Read the model definition and answer for the solid it produces. Units are mm, in the model's axes. A direction names the side the tool comes from. Coordinates: 2 decimals unless noted, no trailing zeros. Write each loop counter-clockwise with the first axis right and the second up, starting at its lowest first coordinate (ties: lowest second). Pieces come first, ordered by that corner, then holes.
(1) The part is cut by section B-B, the plane x = 89. Determine the outline of the cut face in (y, z).
(2) Which of the six approach directions +Z, -Z, +X, -X, +Y, -Y give full straight-line access (tool end or side, diameter ignored) to faces 4 (the flat face through (64, 34, 8)), 5 (the cylindrical face through (112.48, 60, 3.67)), 6 (the cylindrical face through (119.96, 38.81, 3.94))?
(3) Determine the mould class of faces 1 (the cylindrical face through (6.467, 1.862, 3.944)), 2 (the cylindrical face through (22.11, 60, 5.34)), 3 (the flat face through (20, 49.862, 4)) for opening direction Y: pulls with the +Y half, pulls with the -Y half, needs draft (parallel to the pull), parting line crosses it, or undercut.
(4) Given pin 1 (4.5 mm diameter, centred on x = 50, z = 4, fed in from +Y), flat-ended and moving along its own axis, determine where the tip first touches the part or whether it passes through.
(5) The part is cut by section C-C, the plane z = 4. State how many separate pieces and enclosed holes the cut face has, and give its area (3 significant figures).
(6) The part is cut by section A-A, the plane x = 123.5. Determine the outline of the cut face in (y, z), and give its area (3 significant figures).
(7) Straight lines are drawn through the part: line 1 along Y through (x, z) = (65, 2.5); line 2 along X through (y, z) = (7.5, 3.5); line 3 along X through (y, z) = (57.75, 4). For each, find the intervals that lie inside material, in ascending order.
(8) The part is cut by section D-D, the plane x = 50. Determine the outline of the cut face in (y, z), and give its area (3 significant figures).
```python
from build123d import *

# Parameters (mm, degrees)
BOSS_EXTRU_1_DEPTH       = 8
ESQUISSE2_W              = 5.5
ESQUISSE2_H              = 8
ESQUISSE2_W_2            = 6
ENL_V_MAT_EXTRU_1_DEPTH  = 10
ESQUISSE9_R              = 2.5
ENL_V_MAT_EXTRU_6_DEPTH  = 20
ESQUISSE10_R             = 3
ENL_V_MAT_EXTRU_7_DEPTH  = 148.799418472
ENL_V_MAT_EXTRU_12_DEPTH = 148.799418472
ENL_V_MAT_EXTRU_13_DEPTH = 148.799418472


with BuildPart() as part:
    # Esquisse1 → Boss.-Extru.1 (new body)
    with BuildSketch(Plane.XY):
        with BuildLine():
            Line((4, -2.138221462), (126, -2.138221462))
            ThreePointArc((126, -2.138221462), (128.828427125, -0.966648586), (130, 1.861778538))
            Line((130, 1.861778538), (130, 17.861778538))
            Line((130, 17.861778538), (130, 65.861778538))
            ThreePointArc((130, 65.861778538), (128.828427125, 68.690205663), (126, 69.861778538))
            Line((126, 69.861778538), (4, 69.861778538))
            ThreePointArc((4, 69.861778538), (1.171572875, 68.690205663), (0, 65.861778538))
            Line((0, 65.861778538), (0, 17.861778538))
            Line((0, 17.861778538), (0, 1.861778538))
            ThreePointArc((0, 1.861778538), (1.171572875, -0.966648586), (4, -2.138221462))
        make_face()
    extrude(amount=BOSS_EXTRU_1_DEPTH)

    # Esquisse2 → Enlèv. mat.-Extru.1 (cut)
    with BuildSketch(Plane.XY.offset(8)):
        with Locations((13.75, 10.861778538)):
            Rectangle(ESQUISSE2_W, ESQUISSE2_H)
        with Locations((56.5, 10.861778538)):
            Rectangle(ESQUISSE2_W_2, ESQUISSE2_H)
        with Locations((73.5, 10.861778538)):
            Rectangle(ESQUISSE2_W_2, ESQUISSE2_H)
        with Locations((116.25, 10.861778538)):
            Rectangle(ESQUISSE2_W, ESQUISSE2_H)
    extrude(amount=-ENL_V_MAT_EXTRU_1_DEPTH, mode=Mode.SUBTRACT)

    # Esquisse9 → Enlèv. mat.-Extru.6 (cut)
    with BuildSketch(Plane(origin=(0, 69.861778538, 0), x_dir=(1, 0, 0), z_dir=(0, 1, 0))):
        with Locations(Location((20, -4, 0), (0, 0, 270))):
            Circle(ESQUISSE9_R)
        with Locations(Location((50, -4, 0), (0, 0, 270))):
            Circle(ESQUISSE9_R)
        with Locations(Location((80, -4, 0), (0, 0, 270))):
            Circle(ESQUISSE9_R)
        with Locations(Location((110, -4, 0), (0, 0, 270))):
            Circle(ESQUISSE9_R)
    extrude(amount=-ENL_V_MAT_EXTRU_6_DEPTH, mode=Mode.SUBTRACT)

    # Esquisse10 → Enlèv. mat.-Extru.7 (cut, through all)
    with BuildSketch(Plane.XY.offset(8)):
        with Locations((41, 62.861778538)):
            Circle(ESQUISSE10_R)
        with Locations(Location((41, 27.861778538, 0), (0, 0, 180))):
            Circle(ESQUISSE10_R)
        with Locations((65, 62.861778538)):
            Circle(ESQUISSE10_R)
        with Locations(Location((65, 27.861778538, 0), (0, 0, 180))):
            Circle(ESQUISSE10_R)
        with Locations((89, 62.861778538)):
            Circle(ESQUISSE10_R)
        with Locations(Location((89, 27.861778538, 0), (0, 0, 180))):
            Circle(ESQUISSE10_R)
    extrude(amount=-ENL_V_MAT_EXTRU_7_DEPTH, mode=Mode.SUBTRACT)

    # Esquisse18 → Enlèv. mat.-Extru.12 (cut, through all)
    with BuildSketch(Plane(origin=(0, 0, 0), x_dir=(-1, 0, 0), z_dir=(0, 0, -1))):
        with BuildLine():
            Line((-125, 3.361778538), (-125, 5.361778538))
            ThreePointArc((-125, 5.361778538), (-123.5, 6.861778538), (-122, 5.361778538))
            Line((-122, 5.361778538), (-122, 3.361778538))
            ThreePointArc((-122, 3.361778538), (-123.5, 1.861778538), (-125, 3.361778538))
        make_face()
        with BuildLine():
            Line((-125, 16.361778538), (-125, 14.361778538))
            ThreePointArc((-125, 14.361778538), (-123.5, 12.861778538), (-122, 14.361778538))
            Line((-122, 14.361778538), (-122, 16.361778538))
            ThreePointArc((-122, 16.361778538), (-123.5, 17.861778538), (-125, 16.361778538))
        make_face()
        with BuildLine():
            Line((-8, 3.361778538), (-8, 5.361778538))
            ThreePointArc((-8, 5.361778538), (-6.5, 6.861778538), (-5, 5.361778538))
            Line((-5, 5.361778538), (-5, 3.361778538))
            ThreePointArc((-5, 3.361778538), (-6.5, 1.861778538), (-8, 3.361778538))
        make_face()
        with BuildLine():
            Line((-8, 16.361778538), (-8, 14.361778538))
            ThreePointArc((-8, 14.361778538), (-6.5, 12.861778538), (-5, 14.361778538))
            Line((-5, 14.361778538), (-5, 16.361778538))
            ThreePointArc((-5, 16.361778538), (-6.5, 17.861778538), (-8, 16.361778538))
        make_face()
    extrude(amount=-ENL_V_MAT_EXTRU_12_DEPTH, mode=Mode.SUBTRACT)

    # Esquisse21 → Enlèv. mat.-Extru.13 (cut, through all)
    with BuildSketch(Plane(origin=(0, 0, 0), x_dir=(-1, 0, 0), z_dir=(0, 0, -1))):
        with BuildLine():
            Line((-122, 40.808238571), (-122, 43.808238571))
            ThreePointArc((-122, 43.808238571), (-120, 45.808238571), (-118, 43.808238571))
            Line((-118, 43.808238571), (-118, 40.808238571))
            ThreePointArc((-118, 40.808238571), (-120, 38.808238571), (-122, 40.808238571))
        make_face()
        with BuildLine():
            Line((-122, 53.808238571), (-122, 50.808238571))
            ThreePointArc((-122, 50.808238571), (-120, 48.808238571), (-118, 50.808238571))
            Line((-118, 50.808238571), (-118, 53.808238571))
            ThreePointArc((-118, 53.808238571), (-120, 55.808238571), (-122, 53.808238571))
        make_face()
        with BuildLine():
            Line((-12, 40.808238571), (-12, 43.808238571))
            ThreePointArc((-12, 43.808238571), (-10, 45.808238571), (-8, 43.808238571))
            Line((-8, 43.808238571), (-8, 40.808238571))
            ThreePointArc((-8, 40.808238571), (-10, 38.808238571), (-12, 40.808238571))
        make_face()
        with BuildLine():
            Line((-12, 53.808238571), (-12, 50.808238571))
            ThreePointArc((-12, 50.808238571), (-10, 48.808238571), (-8, 50.808238571))
            Line((-8, 50.808238571), (-8, 53.808238571))
            ThreePointArc((-8, 53.808238571), (-10, 55.808238571), (-12, 53.808238571))
        make_face()
    extrude(amount=-ENL_V_MAT_EXTRU_13_DEPTH, mode=Mode.SUBTRACT)


solid = part.part
```
Computed:
1. outline: (-2.14, 0) - (24.86, 0) - (24.86, 8) - (-2.14, 8) - close; (30.86, 0) - (59.86, 0) - (59.86, 8) - (30.86, 8) - close; (65.86, 0) - (69.86, 0) - (69.86, 8) - (65.86, 8) - close
2. face 4: +Z, +X, -X, +Y, -Y
2. face 5: +Y
2. face 6: +Z, -Z
3. face 1: undercut
3. face 2: needs draft
3. face 3: pulls with the +Y half
4. pin 1: stops at y = 49.86
5. separate pieces: 1
5. enclosed holes: 18
5. area: 8,440 mm2
6. outline: (-2.14, 0) - (1.86, 0) - (1.86, 8) - (-2.14, 8) - close; (6.86, 0) - (12.86, 0) - (12.86, 8) - (6.86, 8) - close; (17.86, 0) - (69.86, 0) - (69.86, 8) - (17.86, 8) - close
6. area: 496 mm2
7. line 1: y = -2.14 to 24.86, 30.86 to 59.86, 65.86 to 69.86
7. line 2: x = 0 to 11, 16.5 to 53.5, 59.5 to 70.5, 76.5 to 113.5, 119 to 130
7. line 3: x = 0 to 17.5, 22.5 to 47.5, 52.5 to 77.5, 82.5 to 107.5, 112.5 to 130
8. outline: (-2.14, 0) - (69.86, 0) - (69.86, 1.5) - (49.86, 1.5) - (49.86, 6.5) - (69.86, 6.5) - (69.86, 8) - (-2.14, 8) - close
8. area: 476 mm2
